Source: CAD feature listing. Evaluate the final solid. Frame: model axes, mm. A direction names the side the tool comes from. Give positions to 0.01 mm unless a question says otherwise; leave off trailing zeros. Order: outer loops, then holes, each group sorted by start corner. A loop starts at its lowest first (then second) coordinate and runs counter-clockwise, first axis right, second up. Notation, with made-up numbers: (7.25, 82) -> (27.25, 82) arc R17 ccw to (27.25, 94) -> close; hole circle Ø11 at (18.5, 9.5). An arc over 180 degrees is marked (long way). Answer in a Markdown table with one row per item.
```python
from build123d import *

# Parameters (mm, degrees)
SKETCH1_W                      = 10
SKETCH1_H                      = 20
SKETCH1_R                      = 1.175
BOSS_EXTRUDE1_DEPTH            = 3
CBORE_FOR_M2_SHCS1_D           = 2.4
CBORE_FOR_M2_SHCS1_CBORE_D     = 4.4
CBORE_FOR_M2_SHCS1_CBORE_DEPTH = 2
SKETCH6_W                      = 10
SKETCH6_H                      = 3
BOSS_EXTRUDE2_DEPTH            = 20
SKETCH8_W                      = 3
SKETCH8_H                      = 20
BOSS_EXTRUDE3_DEPTH            = 15
SKETCH9_R                      = 1.75
CUT_EXTRUDE1_DEPTH             = 45.418464629
FILLET1_R                      = 1
FILLET2_R                      = 1


with BuildPart() as part:
    # Sketch1 → Boss-Extrude1 (new body)
    with BuildSketch(Plane(origin=(0, 0, 0), x_dir=(1, 0, 0), z_dir=(0, 1, 0))):
        with Locations((5, 10)):
            Rectangle(SKETCH1_W, SKETCH1_H)
        with Locations(Location((6.5, 5.25, 0), (0, 0, 270))):
            Circle(SKETCH1_R, mode=Mode.SUBTRACT)
        with Locations(Location((6.5, 14.75, 0), (0, 0, 270))):
            Circle(SKETCH1_R, mode=Mode.SUBTRACT)
    extrude(amount=BOSS_EXTRUDE1_DEPTH)

    # CBORE for M2 SHCS1 (through all)
    with Locations(Plane(origin=(0, 3, 0), x_dir=(1, 0, 0), z_dir=(0, 1, 0))):
        with Locations((6.5, 14.75), (6.5, 5.25)):
            CounterBoreHole(CBORE_FOR_M2_SHCS1_D / 2, CBORE_FOR_M2_SHCS1_CBORE_D / 2, CBORE_FOR_M2_SHCS1_CBORE_DEPTH)

    # Sketch6 → Boss-Extrude2 (add)
    with BuildSketch(Plane(origin=(0, 0, -20), x_dir=(-1, 0, 0), z_dir=(0, 0, -1))):
        with Locations((-5, 1.5)):
            Rectangle(SKETCH6_W, SKETCH6_H)
    extrude(amount=BOSS_EXTRUDE2_DEPTH)

    # Sketch8 → Boss-Extrude3 (add)
    with BuildSketch(Plane(origin=(0, 3, 0), x_dir=(1, 0, 0), z_dir=(0, 1, 0))):
        with Locations((1.5, 30)):
            Rectangle(SKETCH8_W, SKETCH8_H)
    extrude(amount=BOSS_EXTRUDE3_DEPTH)

    # Sketch9 → Cut-Extrude1 (cut, through all)
    with BuildSketch(Plane(origin=(3, 0, 0), x_dir=(0, 0, -1), z_dir=(1, 0, 0))):
        with Locations((35, 13)):
            Circle(SKETCH9_R)
    extrude(amount=-CUT_EXTRUDE1_DEPTH, mode=Mode.SUBTRACT)

    # Fillet1
    fillet1_edges = [part.edges().sort_by_distance(p)[0] for p in [
        (1.5, 3, -20),
        (3, 3, -30),
    ]]
    fillet(fillet1_edges, radius=FILLET1_R)

    # Fillet2
    fillet2_edges = [part.edges().sort_by_distance(p)[0] for p in [
        (0, 0, -20),
    ]]
    fillet(fillet2_edges, radius=FILLET2_R)


solid = part.part
```
(1) Pull-direction query (X, two-part tool) for faces 6 (the cylindrical face through (7.7, 0.5, -5.3)), 7 (the flat face through (1, 11, -20)), 8 (the flat face through (0, 9, -29)), 9 (the cylindrical face through (6.76, 0.49, -13.58)); classes: +X half, -X half, draft (parallel to the pull), parting line (faces both ways), or undercut.
A:
| item | result |
|---|---|
| face 6 | undercut |
| face 7 | draft |
| face 8 | -X half |
| face 9 | undercut |
(2) Section query D-D (z = -35). Return the cut outline in (x, y), plus the area to 3 significant figures.
A:
| item | result |
|---|---|
| outline | (0, 1) arc R1 ccw to (1, 0) -> (10, 0) -> (10, 3) -> (4, 3) arc R1 cw to (3, 4) -> (3, 11.25) -> (0, 11.25) -> close; (0, 14.75) -> (3, 14.75) -> (3, 18) -> (0, 18) -> close |
| area | 64.5 mm^2 |
(3) Section query B-B (z = -5.25). Return the cut outline in (x, y), plus the area to 3 significant figures.
A:
| item | result |
|---|---|
| outline | (0, 1) arc R1 ccw to (1, 0) -> (5.3, 0) -> (5.3, 1) -> (4.3, 1) -> (4.3, 3) -> (0, 3) -> close; (7.7, 0) -> (10, 0) -> (10, 3) -> (8.7, 3) -> (8.7, 1) -> (7.7, 1) -> close |
| area | 18.6 mm^2 |
(4) First-contact query: pin 1 Ø1.5 at (x, y) = (2, 7.5) entering from +Z; pin 2 Ø2 at (x, z) = (7, -14.5) entering from +Y; pin 3 Ø5 at (x, z) = (6.5, -14.75) entering from -Y; pin 4 Ø1.5 at (y, z) = (10, -32) entering from +X. Flat tips, straight axial feed; report the tip coordinate or a pass-through.
A:
| item | result |
|---|---|
| pin 1 | stops at z = -20 |
| pin 2 | stops at y = 1 |
| pin 3 | stops at y = 0 |
| pin 4 | stops at x = 3 |
(5) Section query C-C (x = 1.5). Return the cut outline in (y, z), plus the area to 3 significant figures.
A:
| item | result |
|---|---|
| outline | (0, -40) -> (18, -40) -> (18, -20) -> (4, -20) arc R1 cw to (3, -19) -> (3, 0) -> (0, 0) -> close; hole circle Ø3.5 at (13, -35) |
| area | 411 mm^2 |
(6) Access query for faces 1 (the flat face through (6, 0, -20)), 2 (the cylindrical face through (1.584, 3.301, -19.715)), 3 (the flat face through (3, 11, -30)), 4 (the cylindrical face through (8.532, 2.014, -13.907)), 5 (the flat face through (6, 3, -20)). Directions: +Z, -Z, +X, -X, +Y, -Y. A direction counts if a zero-diameter tool reaches every point of the face in a straight line with its end or side. Return the directions, or none.
A:
| item | result |
|---|---|
| face 1 | +Z, -Z, +X, -X, -Y |
| face 2 | +Z, +X, -X, +Y |
| face 3 | +Z, -Z, +X, +Y |
| face 4 | +Y |
| face 5 | +Z, +X, +Y |
(7) Section query A-A (x = 6.5). Return the cut outline in (y, z), plus the area to 3 significant figures.
A:
| item | result |
|---|---|
| outline | (0, -40) -> (3, -40) -> (3, -16.95) -> (1, -16.95) -> (1, -15.95) -> (0, -15.95) -> close; (0, -13.55) -> (1, -13.55) -> (1, -12.55) -> (3, -12.55) -> (3, -7.45) -> (1, -7.45) -> (1, -6.45) -> (0, -6.45) -> close; (0, -4.05) -> (1, -4.05) -> (1, -3.05) -> (3, -3.05) -> (3, 0) -> (0, 0) -> close |
| area | 97.6 mm^2 |
(8) Ray query, probe 1 along Z at (x, y) = (6.5, 0.45); probe 2 along Y at (x, z) = (9.25, -3.5). Return the intervals inside material, ascending.
A:
| item | result |
|---|---|
| probe 1 | z = -40 to -15.95, -13.55 to -6.45, -4.05 to 0 |
| probe 2 | y = 0 to 3 |
